Design review of the part built by this model. Coordinates are the model's own, in mm. Face numbers are marked on the shaded views. A direction names the side the tool comes from. Give positions to 0.01 mm unless a question says otherwise; leave off trailing zeros. Order: outer loops, then holes, each group sorted by start corner. A loop starts at its lowest first (then second) coordinate and runs counter-clockwise, first axis right, second up.
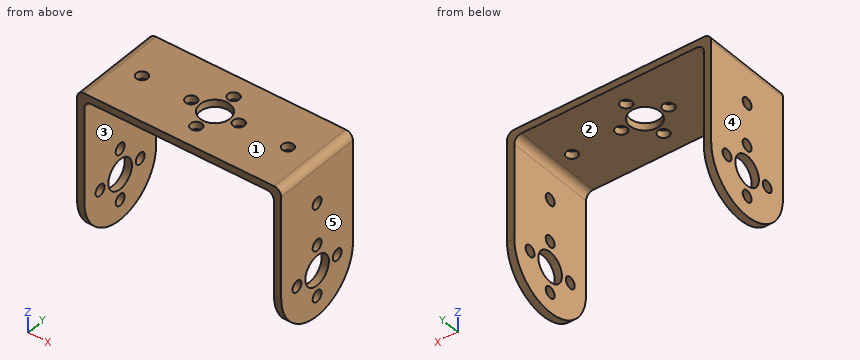
```python
from build123d import *

# Parameters (mm, degrees)
SKETCH_1_W            = 56
SKETCH_1_H            = 25
EXTRUDE_1_DEPTH       = 2
EXTRUDE_START         = -2
EXTRUDE_2_OUTLINE_R   = 1.55
EXTRUDE_2_OUTLINE_R_2 = 4.1
EXTRUDE_2_DEPTH       = 2
SKETCH_3_R            = 1.55
SKETCH_3_R_2          = 4.1
CUT_EXTRUDE_1_DEPTH   = 2
FILLET_1_R            = 2


# Read off the part's stored shape, not the designer's step: 凸台-拉伸2
with BuildPart() as part:
    # 草图1 → 凸台-拉伸1 (new body)
    with BuildSketch(Plane.XY):
        Rectangle(SKETCH_1_W, SKETCH_1_H)
    extrude(amount=EXTRUDE_1_DEPTH)

    # 凸台-拉伸2 outline → 凸台-拉伸2 (add)
    with BuildSketch(Plane(origin=(28, 0, 0), x_dir=(0, 0, -1), z_dir=(1, 0, 0)).offset(EXTRUDE_START)):
        with BuildLine():
            Line((0, -12.5), (28, -12.5))
            ThreePointArc((28, -12.5), (40.5, 0), (28, 12.5))
            Line((28, 12.5), (0, 12.5))
            Line((0, 12.5), (0, -12.5))
        make_face()
        with Locations((28, -7)):
            Circle(EXTRUDE_2_OUTLINE_R, mode=Mode.SUBTRACT)
        with Locations((9.5, 0)):
            Circle(EXTRUDE_2_OUTLINE_R, mode=Mode.SUBTRACT)
        with Locations((21, 0)):
            Circle(EXTRUDE_2_OUTLINE_R, mode=Mode.SUBTRACT)
        with Locations((28, 0)):
            Circle(EXTRUDE_2_OUTLINE_R_2, mode=Mode.SUBTRACT)
        with Locations((35, 0)):
            Circle(EXTRUDE_2_OUTLINE_R, mode=Mode.SUBTRACT)
        with Locations((28, 7)):
            Circle(EXTRUDE_2_OUTLINE_R, mode=Mode.SUBTRACT)
    extrude_2 = extrude(amount=EXTRUDE_2_DEPTH)

    # 镜向2: 凸台-拉伸2 across plane
    add(extrude_2.mirror(Plane.ZY))

    # 草图3 → 切除-拉伸1 (cut)
    with BuildSketch(Plane.XY.offset(2)):
        with Locations((-20, 0)):
            Circle(SKETCH_3_R)
        with Locations((-6.5, 0)):
            Circle(SKETCH_3_R)
        with Locations((6.5, 0)):
            Circle(SKETCH_3_R)
        with Locations((0, -6.5)):
            Circle(SKETCH_3_R)
        Circle(SKETCH_3_R_2)
        with Locations((0, 6.5)):
            Circle(SKETCH_3_R)
        with Locations((20, 0)):
            Circle(SKETCH_3_R)
    extrude(amount=-CUT_EXTRUDE_1_DEPTH, mode=Mode.SUBTRACT)

    # 圆角1
    fillet_1_edges = [part.edges().sort_by_distance(p)[0] for p in [
        (-28, 0, 2),
        (26, 0, 0),
        (-26, 0, 0),
        (28, 0, 2),
    ]]
    fillet(fillet_1_edges, radius=FILLET_1_R)


solid = part.part
```
1. Take a section at D-D (y = 0.75). State how many separate pieces and enclosed holes the cut face has, then the cut area to 3 significant figures.
Recorded:
separate pieces: 14
enclosed holes: 0
area: 171 mm2
2. Take a section at A-A (z = -21). State the section outline as (x, y) points.
Recorded:
outline: (-28, -12.5) - (-26, -12.5) - (-26, -1.55) - (-28, -1.55) - close; (-28, 1.55) - (-26, 1.55) - (-26, 12.5) - (-28, 12.5) - close; (26, -12.5) - (28, -12.5) - (28, -1.55) - (26, -1.55) - close; (26, 1.55) - (28, 1.55) - (28, 12.5) - (26, 12.5) - close
3. Machinability: for the marked faces 1 and 2, which of the approach directions +Z, -Z, +X, -X, +Y, -Y give a long, thin tool a straight path to every point of the face, cutting with its end or side? Answer none if there is none.
Recorded:
face 1: +Z, +X, -X, +Y, -Y
face 2: -Z, +Y, -Y
4. Take a section at C-C (x = 16.5). State the section outline as (y, z) points, then the cut area to 3 significant figures.
Recorded:
outline: (-12.5, 0) - (12.5, 0) - (12.5, 2) - (-12.5, 2) - close
area: 50.0 mm2
5. Draft analysis for pull direction X (two halves, no side actions). For the marked faces 3, 4 and 5, state which applies: pulls with the +X half, pulls with the -X half, needs draft (parallel to the pull), parting line crosses it, or undercut.
Recorded:
face 3: undercut
face 4: pulls with the -X half
face 5: pulls with the +X half
6. For pin 1 (2.5 mm diameter, centred on y = 0, z = -21, fed in from +X); pin 2 (3.5 mm diameter, centred on x = 6.5, y = 0, fed in from -Z), all flat-tipped, find the tip position at first contact; note any pin that passes through.
Recorded:
pin 1: passes through
pin 2: stops at z = 0
7. For line 1 along Y through (x, z) = (27, -28); line 2 along X through (y, z) = (-5, -5.5); line 3 along Z through (x, y) = (9.5, -7.25), list the stretches that pass through material, from the lowest coordinate up.
Recorded:
line 1: y = -12.5 to -8.55, -5.45 to -4.1, 4.1 to 5.45, 8.55 to 12.5
line 2: x = -28 to -26, 26 to 28
line 3: z = 0 to 2
8. Take a section at B-B (x = -6.5). State the section outline as (y, z) points, then the cut area to 3 significant figures.
Recorded:
outline: (-12.5, 0) - (-1.55, 0) - (-1.55, 2) - (-12.5, 2) - close; (1.55, 0) - (12.5, 0) - (12.5, 2) - (1.55, 2) - close
area: 43.8 mm2
